```python
from build123d import *

# Parameters (mm, degrees)
F0_W      = 20
F0_H      = 56
F1_DEPTH  = 5
F2_W      = 20
F2_H      = 10
F3_DEPTH  = 45
F5_D      = 6.528
F7_DEPTH  = 20
F9_DEPTH  = 45
F10_DEPTH = 50.001


with BuildPart() as f1:
    # F0 (on Top) → F1 (new body)
    with BuildSketch(Plane.XY):
        with Locations((-5.1124608144, 7.0487826013)):
            Rectangle(F0_W, F0_H)
    extrude(amount=F1_DEPTH)

    # F2 (on face) → F3 (join)
    with BuildSketch(Plane.XY.offset(5)):
        with Locations((-5.1124608144, -15.9512173987)):
            Rectangle(F2_W, F2_H)
    extrude(amount=F3_DEPTH)

    # F5 (through all)
    with Locations(Plane(origin=(0, 0, 0), x_dir=(1, 0, 0), z_dir=(0, 0, -1))):
        with Locations((-5.1124608144, 2.9512173987)):
            Hole(F5_D / 2)

    # F6 (on face) → F7 (cut, through all)
    with BuildSketch(Plane(origin=(-15.1124608144, 0, 0), x_dir=(0, -1, 0), z_dir=(-1, 0, 0))):
        Polygon((-33.0487826013, 5), (-35.0487826013, 5), (-34.0487826013, 4), align=None)
        Polygon((-31.0487826013, 5), (-33.0487826013, 5), (-32.0487826013, 4), align=None)
        Polygon((-29.0487826013, 5), (-31.0487826013, 5), (-30.0487826013, 4), align=None)
        Polygon((-27.0487826013, 5), (-29.0487826013, 5), (-28.0487826013, 4), align=None)
        Polygon((-25.0487826013, 5), (-27.0487826013, 5), (-26.0487826013, 4), align=None)
        Polygon((-23.0487826013, 5), (-25.0487826013, 5), (-24.0487826013, 4), align=None)
        Polygon((-21.0487826013, 5), (-23.0487826013, 5), (-22.0487826013, 4), align=None)
        Polygon((-19.0487826013, 5), (-21.0487826013, 5), (-20.0487826013, 4), align=None)
        Polygon((-17.0487826013, 5), (-19.0487826013, 5), (-18.0487826013, 4), align=None)
        Polygon((-15.0487826013, 5), (-17.0487826013, 5), (-16.0487826013, 4), align=None)
        Polygon((-13.0487826013, 5), (-15.0487826013, 5), (-14.0487826013, 4), align=None)
        Polygon((-12.0487826013, 4), (-11.0487826013, 5), (-13.0487826013, 5), align=None)
        Polygon((-10.0487826013, 4), (-9.0487826013, 5), (-11.0487826013, 5), align=None)
        Polygon((-8.0487826013, 4), (-7.0487826013, 5), (-9.0487826013, 5), align=None)
        Polygon((-6.0487826013, 4), (-5.0487826013, 5), (-7.0487826013, 5), align=None)
        Polygon((-4.0487826013, 4), (-3.0487826013, 5), (-5.0487826013, 5), align=None)
    extrude(amount=-F7_DEPTH, mode=Mode.SUBTRACT)

    # F8 (on face) → F9 (cut)
    with BuildSketch(Plane.XY.offset(50)):
        Polygon((-1.6124608144, -10.9512173987), (-8.6124608144, -10.9512173987), (-12.1124608144, -15.4354041442), (1.8875391856, -15.4354041442), align=None)
    extrude(amount=-F9_DEPTH, mode=Mode.SUBTRACT)

    # F10 (cut, through all): a face of the model
    f10_faces = [f1.faces().sort_by_distance(p)[0] for p in [
        (-5.1124608144, -16.7236905936, 50),
    ]]
    extrude(f10_faces, amount=-F10_DEPTH, mode=Mode.SUBTRACT)


solid = f1.part
```
Design review of the part built by this model. Coordinates are the model's own, in mm. A direction names the side the tool comes from. Coordinates: 2 decimals unless noted, no trailing zeros. Order: outer loops, then holes, each group sorted by start corner. A loop starts at its lowest first (then second) coordinate and runs counter-clockwise, first axis right, second up.
1) Wall thickness on line 1 along X through (y, z) = (-3, 0.4); line 2 along Y through (x, z) = (4, 2.85); line 3 along Y through (x, z) = (-7, 3.15): over which ranges is each line inside the solid? List them lowest first.
2) For faces 1 (the flat face through (-5.25, 21.56, 4.49)), 2 (the flat face through (-10.338, -13.162, 2.535)), 3 (the cylindrical face through (-4.405, 0.235, 2.535)), 4 (the flat face through (0.16, -13.22, 2.53)), list the 3-axis set-ups (+Z, -Z, +X, -X, +Y, -Y) from which the entire face can be reached by the end or side of a thin tool; tool diameter is ignored.
3) Take a section at A-A, the plane y = -2. Give the boundary of the cut face in (x, z).
4) Take a section at B-B, the plane z = 3.2. Give the boundary of the cut face in (x, y).
5) Take a section at C-C, the plane y = 19.5. Give the boundary of the cut face in (x, z), and give its area (3 significant figures).
6) Mouldability with a two-part tool opening along Y and no side actions: class faces 5 (the flat face through (-5, -15.435, 3)), 6 (the flat face through (-5.25, 5.56, 4.49)), 7 (the flat face through (-5, 10, 0)) as +Y half, -Y half, draft (parallel to the pull), parting line (faces both ways), or undercut.
Returned:
1. line 1: x = -15.11 to -8.38, -1.85 to 4.89
1. line 2: y = -10.95 to 35.05
1. line 3: y = -15.44 to -5.61, -0.29 to 35.05
2. face 1: +Z, +X, -X
2. face 2: +Z, -Z, -X
2. face 3: +Z, -Z
2. face 4: +Z, -Z, +X
3. outline: (-15.11, 0) - (-8.23, 0) - (-8.23, 5) - (-15.11, 5) - close; (-1.99, 0) - (4.89, 0) - (4.89, 5) - (-1.99, 5) - close
4. outline: (-15.11, -10.95) - (-8.61, -10.95) - (-12.11, -15.44) - (1.89, -15.44) - (-1.61, -10.95) - (4.89, -10.95) - (4.89, 35.05) - (-15.11, 35.05) - close; hole circle Ø6.53 at (-5.11, -2.95)
5. outline: (-15.11, 0) - (4.89, 0) - (4.89, 4.55) - (-15.11, 4.55) - close
5. area: 91.0 mm2
6. face 5: -Y half
6. face 6: undercut
6. face 7: draft
